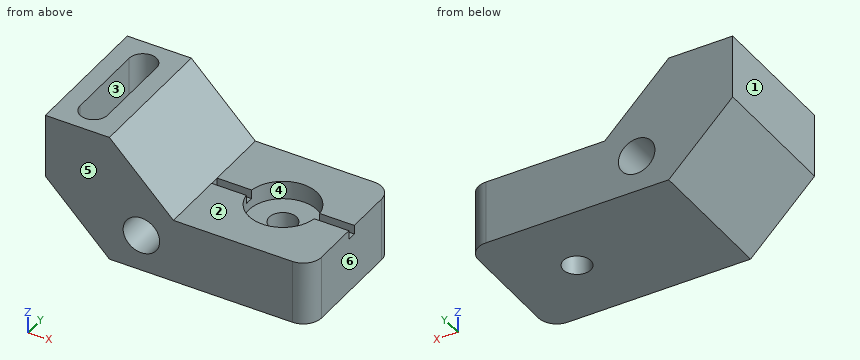
from build123d import *

# Parameters (mm, degrees)
F1_DEPTH       = 76.2
F2_R           = 10.16
F3_DEPTH       = 76.201
F5_DEPTH       = 27.94
F7_D           = 15.24
F7_CBORE_D     = 38.1
F7_CBORE_DEPTH = 10.16
F9_DEPTH       = 76.2
F10_R          = 10.16


with BuildPart() as f1:
    # F0 (on Front) → F1 (new body)
    with BuildSketch(Plane.XZ):
        Polygon((0, 71.12), (0, 35.56), (35.56, 0), (147.32, 0), (147.32, 35.56), (71.12, 35.56), (35.56, 71.12), align=None)
    extrude(amount=F1_DEPTH)

    # F2 (on face) → F3 (cut, through all)
    with BuildSketch(Plane.XZ.offset(76.2)):
        with Locations((53.34, 20.32)):
            Circle(F2_R)
    extrude(amount=-F3_DEPTH, mode=Mode.SUBTRACT)

    # F4 (on face) → F5 (cut)
    with BuildSketch(Plane.XY.offset(71.12)):
        with BuildLine():
            ThreePointArc((25.4, -15.24), (17.78, -7.62), (10.16, -15.24))
            Line((10.16, -15.24), (10.16, -60.96))
            ThreePointArc((10.16, -60.96), (17.78, -68.58), (25.4, -60.96))
            Line((25.4, -60.96), (25.4, -15.24))
        make_face()
    extrude(amount=-F5_DEPTH, mode=Mode.SUBTRACT)

    # F7 (through all)
    with Locations(Plane.XY.offset(35.56)):
        with Locations((109.22, -38.1)):
            CounterBoreHole(F7_D / 2, F7_CBORE_D / 2, F7_CBORE_DEPTH)

    # F8 (on face) → F9 (cut)
    with BuildSketch(Plane.YZ.offset(147.32)):
        Polygon((-35.56, 35.56), (-38.1, 35.56), (-40.64, 35.56), (-40.64, 30.48), (-35.56, 30.48), align=None)
    extrude(amount=-F9_DEPTH, mode=Mode.SUBTRACT)

    # F10
    f10_edges = [f1.edges().sort_by_distance(p)[0] for p in [
        (147.32, 0, 17.78),
        (147.32, -76.2, 17.78),
    ]]
    fillet(f10_edges, radius=F10_R)


solid = f1.part
Design review of the part built by this model. Coordinates are the model's own, in mm. Face numbers are marked on the shaded views. A direction names the side the tool comes from. Round coordinates to 2 decimals unless told otherwise and drop trailing zeros. Loops run counter-clockwise (first coordinate to the right, second up) from the corner with the lowest first, then second, coordinate; pieces in that order, holes last. Notation, with made-up numbers: (-26, 18) - (25, 18) arc R30 cw to (25, 50) - close; hole circle Ø3 at (7.5, -8). An arc over 180 degrees is marked (long way). One line per item, written item: value. Start each with the question number.
1) Insertion check: pin 1 Ø2 at (x, y) = (30, -30.5) entering from -Z; pin 2 Ø18 at (x, y) = (116, -16) entering from +Z; pin 3 Ø1.5 at (x, y) = (54.5, -30) entering from -Z; pin 4 Ø7.5 at (x, y) = (16, -34.5) entering from +Z. Each pin has a flat end and moves straight along its axis. Give the tip position at first contact, or say it passes through.
2) Consider section A-A on z = 20.32. Give the boundary of the cut face in (x, y), then the cut area to 3 significant figures.
3) Consider section D-D on x = 53.34. Give the boundary of the cut face in (y, z).
4) Consider section B-B on x = 109.22. Give the boundary of the cut face in (y, z).
5) Consider section C-C on z = 60.5. Give the boundary of the cut face in (x, y).
6) To check wall thickness, follow L1, parallel to Y at x = 109.22, z = 17.5; L2, parallel to X at y = -38.1, z = 28; L3, parallel to X at y = -45, z = 20. State the ranges of each line that lie inside material, in increasing order. Write a range as from..to.
7) For the marked faces 1, 2 and 3, list the 3-axis set-ups (+Z, -Z, +X, -X, +Y, -Y) from which the entire face can be reached by the end or side of a thin tool; tool diameter is ignored.
8) Draft analysis for pull direction Y (two halves, no side actions). For the marked faces 4, 5 and 6, state which applies: +Y half, -Y half, draft (parallel to the pull), parting line (faces both ways), or undercut.
Reported:
1. pin 1: stops at z = 4.56
1. pin 2: stops at z = 35.56
1. pin 3: stops at z = 0
1. pin 4: stops at z = 43.18
2. outline: (15.24, -76.2) - (43.18, -76.2) - (43.18, 0) - (15.24, 0) - close; (63.5, -76.2) - (137.16, -76.2) arc R10.16 ccw to (147.32, -66.04) - (147.32, -10.16) arc R10.16 ccw to (137.16, 0) - (63.5, 0) - close; hole circle Ø15.24 at (109.22, -38.1)
2. area: 8,290 mm^2
3. outline: (-76.2, 0) - (0, 0) - (0, 10.16) - (-76.2, 10.16) - close; (-76.2, 30.48) - (0, 30.48) - (0, 53.34) - (-76.2, 53.34) - close
4. outline: (-76.2, 0) - (-45.72, 0) - (-45.72, 25.4) - (-57.15, 25.4) - (-57.15, 35.56) - (-76.2, 35.56) - close; (-30.48, 0) - (0, 0) - (0, 35.56) - (-19.05, 35.56) - (-19.05, 25.4) - (-30.48, 25.4) - close
5. outline: (0, -76.2) - (46.18, -76.2) - (46.18, 0) - (0, 0) - close; hole (10.16, -60.96) arc R7.62 ccw to (25.4, -60.96) - (25.4, -15.24) arc R7.62 ccw to (10.16, -15.24) - close
6. L1: y = -76.2..-45.72, -30.48..0
6. L2: x = 7.56..46.69, 59.99..90.17, 128.27..147.32
6. L3: x = 15.56..43.19, 63.49..105.99, 112.45..147.32
7. face 1: +Z, -Z, -X, +Y, -Y
7. face 2: +Z, +X, +Y, -Y
7. face 3: +Z
8. face 4: undercut
8. face 5: -Y half
8. face 6: draft
